from build123d import *

# Parameters (mm, degrees)
ESBO_O2_R                = 20
RESSALTO_EXTRUS_O1_DEPTH = 25
ESBO_O3_R                = 1.25
CORTE_EXTRUS_O1_DEPTH    = 145.913767462


with BuildPart() as part:
    # Esboço2 → Ressalto-extrusão1 (new, symmetric)
    with BuildSketch(Plane(origin=(0, 0, 0), x_dir=(0, 0, -1), z_dir=(1, 0, 0))):
        with BuildLine():
            Line((-50.981554588, -22.5), (29.018445412, -22.5))
            ThreePointArc((29.018445412, -22.5), (49.706343576, -25.409703361), (68.789024491, -33.913043478))
            ThreePointArc((68.789024491, -33.913043478), (130, 0), (68.789024491, 33.913043478))
            ThreePointArc((68.789024491, 33.913043478), (49.706343576, 25.409703361), (29.018445412, 22.5))
            Line((29.018445412, 22.5), (-50.981554588, 22.5))
            Line((-50.981554588, 22.5), (-50.981554588, -22.5))
        make_face()
        with Locations((90, 0)):
            Circle(ESBO_O2_R, mode=Mode.SUBTRACT)
        with BuildLine():
            ThreePointArc((67.339434728, -12.747500993), (72.162673174, -18.916388971), (78.603905138, -23.369403542))
            ThreePointArc((78.603905138, -23.369403542), (79.064417011, -24.706538096), (77.727282457, -25.167049968))
            ThreePointArc((77.727282457, -25.167049968), (70.79057111, -20.371495815), (65.596314323, -13.728077992))
            ThreePointArc((65.596314323, -13.728077992), (65.977586026, -12.36622929), (67.339434728, -12.747500993))
        make_face(mode=Mode.SUBTRACT)
        with BuildLine():
            ThreePointArc((61.238513309, -16.179520491), (67.360315951, -24.009262924), (75.535725753, -29.661166034))
            ThreePointArc((75.535725753, -29.661166034), (75.996237625, -30.998300588), (74.659103071, -31.45881246))
            ThreePointArc((74.659103071, -31.45881246), (65.988213888, -25.464369768), (59.495392903, -17.16009749))
            ThreePointArc((59.495392903, -17.16009749), (59.876664606, -15.798248788), (61.238513309, -16.179520491))
        make_face(mode=Mode.SUBTRACT)
        with BuildLine():
            ThreePointArc((59.495392903, 17.16009749), (59.876664606, 15.798248788), (61.238513309, 16.179520491))
            ThreePointArc((61.238513309, 16.179520491), (67.360315951, 24.009262924), (75.535725753, 29.661166034))
            ThreePointArc((75.535725753, 29.661166034), (75.996237625, 30.998300588), (74.659103071, 31.45881246))
            ThreePointArc((74.659103071, 31.45881246), (65.988213888, 25.464369768), (59.495392903, 17.16009749))
        make_face(mode=Mode.SUBTRACT)
        with BuildLine():
            ThreePointArc((65.596314323, 13.728077992), (65.977586026, 12.36622929), (67.339434728, 12.747500993))
            ThreePointArc((67.339434728, 12.747500993), (72.162673174, 18.916388971), (78.603905138, 23.369403542))
            ThreePointArc((78.603905138, 23.369403542), (79.064417011, 24.706538096), (77.727282457, 25.167049968))
            ThreePointArc((77.727282457, 25.167049968), (70.79057111, 20.371495815), (65.596314323, 13.728077992))
        make_face(mode=Mode.SUBTRACT)
        with BuildLine():
            ThreePointArc((90, -35), (125, 0), (90, 35))
            ThreePointArc((90, 35), (89, 34), (90, 33))
            ThreePointArc((90, 33), (123, 0), (90, -33))
            ThreePointArc((90, -33), (89, -34), (90, -35))
        make_face(mode=Mode.SUBTRACT)
        with BuildLine():
            ThreePointArc((90, -28), (118, 0), (90, 28))
            ThreePointArc((90, 28), (89, 27), (90, 26))
            ThreePointArc((90, 26), (116, 0), (90, -26))
            ThreePointArc((90, -26), (89, -27), (90, -28))
        make_face(mode=Mode.SUBTRACT)
        with BuildLine():
            ThreePointArc((80.278403844, 20.844437344), (74.464540757, 16.960233079), (70.086402165, 11.508632467))
            ThreePointArc((70.086402165, 11.508632467), (70.451835442, 10.142448541), (71.818019368, 10.507881818))
            ThreePointArc((71.818019368, 10.507881818), (75.815450256, 15.485430203), (81.123760031, 19.031877575))
            ThreePointArc((81.123760031, 19.031877575), (81.607361822, 20.360835553), (80.278403844, 20.844437344))
        make_face(mode=Mode.SUBTRACT)
        with BuildLine():
            ThreePointArc((69.641858511, -10.702620013), (73.984708204, -16.507889892), (79.918839161, -20.672933902))
            ThreePointArc((79.918839161, -20.672933902), (81.255973715, -20.21242203), (80.795461843, -18.875287476))
            ThreePointArc((80.795461843, -18.875287476), (75.377342273, -15.072421206), (71.412131684, -9.771957403))
            ThreePointArc((71.412131684, -9.771957403), (70.061663793, -9.352152121), (69.641858511, -10.702620013))
        make_face(mode=Mode.SUBTRACT)
        with BuildLine():
            ThreePointArc((89.378360714, -22.991597696), (112.997899328, -0.310848034), (90, 23))
            ThreePointArc((90, 23), (89, 22), (90, 21))
            ThreePointArc((90, 21), (110.998081995, -0.28381777), (89.432416304, -20.992328331))
            ThreePointArc((89.432416304, -20.992328331), (88.405753826, -21.964935218), (89.378360714, -22.991597696))
        make_face(mode=Mode.SUBTRACT)
    extrude(amount=RESSALTO_EXTRUS_O1_DEPTH, both=True)

    # Esboço3 → Corte-extrusão1 (cut, through all)
    with BuildSketch(Plane.ZY.offset(25)):
        with Locations((25.881554588, 7.5)):
            Circle(ESBO_O3_R)
        with Locations((-9.118445412, 7.5)):
            Circle(ESBO_O3_R)
        with Locations((-9.118445412, -7.5)):
            Circle(ESBO_O3_R)
        with Locations((25.881554588, -7.5)):
            Circle(ESBO_O3_R)
    extrude(amount=-CORTE_EXTRUS_O1_DEPTH, mode=Mode.SUBTRACT)


solid = part.part
CAD build for the part. Positions are in the model's coordinates, mm. A direction names the side the tool comes from. Coordinates: 2 decimals unless noted, no trailing zeros. Loops run counter-clockwise (first coordinate to the right, second up) from the corner with the lowest first, then second, coordinate; pieces in that order, holes last. Notation, with made-up numbers: (-20.75, -33.5) -> (25.25, -33.5) arc R18 cw to (25.25, -3.5) -> close; hole circle Ø6 at (57, -25). An arc over 180 degrees is marked (long way). One line per item, written item: value.
1. Slice it at A-A on y = 0. Write the cut outline in (x, z), and give its area (3 significant figures).
Answers:
outline: (-25, -130) -> (25, -130) -> (25, -125) -> (-25, -125) -> close; (-25, -123) -> (25, -123) -> (25, -118) -> (-25, -118) -> close; (-25, -116) -> (25, -116) -> (25, -113) -> (-25, -113) -> close; (-25, -111) -> (25, -111) -> (25, -110) -> (-25, -110) -> close; (-25, -70) -> (25, -70) -> (25, 50.98) -> (-25, 50.98) -> close
area: 6,750 mm^2
2. Slice it at B-B on z = -104. Give the number of separate pieces and of enclosed holes in the cut face, and give its area (3 significant figures).
Answers:
separate pieces: 8
enclosed holes: 0
area: 1,610 mm^2
3. Flat gauge pins, fed straight in: P1, Ø5, axis at x = -11, z = -27, coming from the -Y side; P2, Ø6, axis at x = -10, z = -61.5, coming from the +Y side. Where does each tip first touch, or does it go through?
Answers:
P1: stops at y = -22.5
P2: stops at y = 31.42
4. Slice it at C-C on z = -25. Write the cut outline in (x, y), and give its area (3 significant figures).
Answers:
outline: (-25, -22.5) -> (25, -22.5) -> (25, 22.5) -> (-25, 22.5) -> close
area: 2,250 mm^2
5. Which spindle directions (+Z, -Z, +X, -X, +Y, -Y) get a long thin tool onto all of the face, cutting with end or side? Do faces 1 (the face through (0.35, -25.33, -49.42)), 2 (the face through (0.35, 18.84, -72.08)). Say none if no direction does.
Answers:
face 1: +Z, +X, -X, -Y
face 2: +X, -X
6. Drill centre lines: line 1 (Z direction, x = -5.5, y = 6); line 2 (Y direction, x = 15, z = -62); line 3 (Y direction, x = 20, z = -119.5). Where is each one in solid material? Low to high. Write a range as [from, to].
Answers:
line 1: z = [-129.55, -124.48], [-122.45, -117.35], [-115.3, -112.2], [-110.12, -109.08], [-70.92, 50.98]
line 2: y = [-30.14, -21], [-17.46, 17.46], [21, 30.14]
line 3: y = [-27.01, -18.83], [-14.79, 14.79], [18.83, 27.01]
7. Pull direction Y, two halves, no side cores. Call faces 3 (the face through (0.35, -16.437, -73.912)), 4 (the face through (0, 0, 50.982)), 5 (the face through (0.35, -1.192, -129.982)): pulls with the +Y half, pulls with the -Y half, needs draft (parallel to the pull), parting line crosses it, or undercut.
Answers:
face 3: undercut
face 4: needs draft
face 5: parting line crosses it
